from build123d import *

# Parameters (mm, degrees)
F0_W         = 16.3
F0_H         = 8.5
F1_DEPTH     = 22
F2_R         = 5.1
F3_DEPTH     = 22
F4_W         = 3
F4_H         = 12.2
F4_W_2       = 9.2
F5_DEPTH     = 40
F6_R         = 2.5
F7_DEPTH     = 22.001
F6_R_2       = 4.25
F8_DEPTH     = 5
F9_T1_DEPTH  = 85
F9_T3_DEPTH  = 36
F9_T5_DEPTH  = 20
F9_S9_W      = 1
F9_S9_H      = 1
F9_T10_DEPTH = 1
F9_S15_W     = 1
F9_S15_H     = 1
F9_T16_DEPTH = 1
F9_S21_W     = 1
F9_S21_H     = 1
F9_T22_DEPTH = 1
F9_S27_W     = 1
F9_S27_H     = 1
F9_T28_DEPTH = 1
F9_S33_W     = 1
F9_S33_H     = 1
F9_T34_DEPTH = 1
F9_S39_W     = 1
F9_S39_H     = 1
F9_T40_DEPTH = 1
F9_S45_W     = 1
F9_S45_H     = 1
F9_T46_DEPTH = 1
F9_S51_W     = 1
F9_S51_H     = 1
F9_T52_DEPTH = 1


# Not quite as in the source:
# - a fillet or chamfer that OpenCascade refuses, or shapes differently, is made with other operations: its cross-section is extruded or revolved along the edge and cut away or added


with BuildPart() as f1:
    # F0 (on Front) → F1 (new body)
    with BuildSketch(Plane.XZ):
        Polygon((-19, 32), (-6.1, 32), (6.1, 32), (19, 32), (19, 54), (-19, 54), align=None)
        with Locations((0, 43)):
            Rectangle(F0_W, F0_H, mode=Mode.SUBTRACT)
        Polygon((-3.1, -20), (-3.1, 20), (-6.1, 20), (-6.1, 32), (-19, 32), (-19, -33), (19, -33), (19, 32), (6.1, 32), (6.1, 20), (3.1, 20), (3.1, -20), align=None)
    extrude(amount=F1_DEPTH)

    # F2 (on face) → F3 (cut, through all)
    with BuildSketch(Plane.XY.offset(54)):
        with Locations((0, -11)):
            Circle(F2_R)
    extrude(amount=-F3_DEPTH, mode=Mode.SUBTRACT)

    # F4 (on face) → F5 (cut)
    with BuildSketch(Plane.XY.offset(20)):
        with Locations((-4.6, -11.319772105)):
            Rectangle(F4_W, F4_H)
        with Locations((1.5, -11.319772105)):
            Rectangle(F4_W_2, F4_H)
    extrude(amount=-F5_DEPTH, mode=Mode.SUBTRACT)

    # F6 (on face) → F7 (cut, through all)
    with BuildSketch(Plane.XZ.offset(22)):
        with Locations((-13, 49)):
            Circle(F6_R)
        with Locations((13, 49)):
            Circle(F6_R)
        with Locations((-13, -27)):
            Circle(F6_R)
        with Locations((13, -27)):
            Circle(F6_R)
    extrude(amount=-F7_DEPTH, mode=Mode.SUBTRACT)

    # F6 (on face) → F8 (cut)
    with BuildSketch(Plane.XZ.offset(22)):
        with Locations((-13, 49)):
            Circle(F6_R_2)
        with Locations((-13, 49)):
            Circle(F6_R, mode=Mode.SUBTRACT)
        with Locations((13, 49)):
            Circle(F6_R_2)
        with Locations((13, 49)):
            Circle(F6_R, mode=Mode.SUBTRACT)
        with Locations((13, -27)):
            Circle(F6_R_2)
        with Locations((13, -27)):
            Circle(F6_R, mode=Mode.SUBTRACT)
        with Locations((-13, -27)):
            Circle(F6_R_2)
        with Locations((-13, -27)):
            Circle(F6_R, mode=Mode.SUBTRACT)
    extrude(amount=-F8_DEPTH, mode=Mode.SUBTRACT)

    # F9: fillet of radius 1 on 12 edges, made by hand

    # F9_s2 → F9_t1 (cut)
    with BuildSketch(Plane.XY.offset(-32)):
        with BuildLine():
            ThreePointArc((18, -22), (18.7071067812, -21.7071067812), (19, -21))
            Line((19, -21), (19, -22))
            Line((19, -22), (18, -22))
        make_face()
        with BuildLine():
            ThreePointArc((-18, -22), (-18.7071067812, -21.7071067812), (-19, -21))
            Line((-19, -21), (-19, -22))
            Line((-19, -22), (-18, -22))
        make_face()
        with BuildLine():
            ThreePointArc((-18, 0), (-18.7071067812, -0.2928932188), (-19, -1))
            Line((-19, -1), (-19, 0))
            Line((-19, 0), (-18, 0))
        make_face()
        with BuildLine():
            ThreePointArc((18, 0), (18.7071067812, -0.2928932188), (19, -1))
            Line((19, -1), (19, 0))
            Line((19, 0), (18, 0))
        make_face()
    extrude(amount=F9_T1_DEPTH, mode=Mode.SUBTRACT)

    # F9_s4 → F9_t3 (cut)
    with BuildSketch(Plane.YZ.offset(-18)):
        with BuildLine():
            ThreePointArc((-22, 53), (-21.7071067812, 53.7071067812), (-21, 54))
            Line((-21, 54), (-22, 54))
            Line((-22, 54), (-22, 53))
        make_face()
        with BuildLine():
            ThreePointArc((-22, -32), (-21.7071067812, -32.7071067812), (-21, -33))
            Line((-21, -33), (-22, -33))
            Line((-22, -33), (-22, -32))
        make_face()
        with BuildLine():
            ThreePointArc((0, 53), (-0.2928932188, 53.7071067812), (-1, 54))
            Line((-1, 54), (0, 54))
            Line((0, 54), (0, 53))
        make_face()
        with BuildLine():
            ThreePointArc((0, -32), (-0.2928932188, -32.7071067812), (-1, -33))
            Line((-1, -33), (0, -33))
            Line((0, -33), (0, -32))
        make_face()
    extrude(amount=F9_T3_DEPTH, mode=Mode.SUBTRACT)

    # F9_s6 → F9_t5 (cut)
    with BuildSketch(Plane.XZ.offset(1)):
        with BuildLine():
            ThreePointArc((19, -32), (18.7071067812, -32.7071067812), (18, -33))
            Line((18, -33), (19, -33))
            Line((19, -33), (19, -32))
        make_face()
        with BuildLine():
            ThreePointArc((18, 54), (18.7071067812, 53.7071067812), (19, 53))
            Line((19, 53), (19, 54))
            Line((19, 54), (18, 54))
        make_face()
        with BuildLine():
            ThreePointArc((-18, 54), (-18.7071067812, 53.7071067812), (-19, 53))
            Line((-19, 53), (-19, 54))
            Line((-19, 54), (-18, 54))
        make_face()
        with BuildLine():
            ThreePointArc((-19, -32), (-18.7071067812, -32.7071067812), (-18, -33))
            Line((-18, -33), (-19, -33))
            Line((-19, -33), (-19, -32))
        make_face()
    extrude(amount=F9_T5_DEPTH, mode=Mode.SUBTRACT)


with BuildPart() as f9_tool8:
    # F9_s9 → F9_t10 (new body)
    with BuildSketch(Plane.XZ.offset(21)):
        with Locations((18.5, -32.5)):
            Rectangle(F9_S9_W, F9_S9_H)
    extrude(amount=F9_T10_DEPTH)

    # F9_s11 → F9_t12 (revolve, cut)
    with BuildSketch(Plane(origin=(18, -21, -32), x_dir=(-0.7071067812, 0, 0.7071067812), z_dir=(0.7071067812, 0, 0.7071067812))):
        with BuildLine():
            ThreePointArc((0, -1), (1, 0), (0, 1))
            Line((0, 1), (0, -1))
        make_face()
    revolve(axis=Axis((18, -21, -32), (0, -1, 0)), mode=Mode.SUBTRACT)


with BuildPart() as f1_1:
    add(f1.part)

    # F9_t7: cut F9_tool8
    add(f9_tool8.part, mode=Mode.SUBTRACT)


with BuildPart() as f9_tool14:
    # F9_s15 → F9_t16 (new body)
    with BuildSketch(Plane.XY.offset(53)):
        with Locations((18.5, -21.5)):
            Rectangle(F9_S15_W, F9_S15_H)
    extrude(amount=F9_T16_DEPTH)

    # F9_s17 → F9_t18 (revolve, cut)
    with BuildSketch(Plane(origin=(18, -21, 53), x_dir=(-0.7071067812, 0.7071067812, 0), z_dir=(0.7071067812, 0.7071067812, 0))):
        with BuildLine():
            ThreePointArc((0, -1), (1, 0), (0, 1))
            Line((0, 1), (0, -1))
        make_face()
    revolve(axis=Axis((18, -21, 53), (0, 0, 1)), mode=Mode.SUBTRACT)


with BuildPart() as f1_2:
    add(f1_1.part)

    # F9_t13: cut F9_tool14
    add(f9_tool14.part, mode=Mode.SUBTRACT)


with BuildPart() as f9_tool20:
    # F9_s21 → F9_t22 (new body)
    with BuildSketch(Plane.XY.offset(53)):
        with Locations((-18.5, -21.5)):
            Rectangle(F9_S21_W, F9_S21_H)
    extrude(amount=F9_T22_DEPTH)

    # F9_s23 → F9_t24 (revolve, cut)
    with BuildSketch(Plane(origin=(-18, -21, 53), x_dir=(0.7071067812, 0.7071067812, 0), z_dir=(0.7071067812, -0.7071067812, 0))):
        with BuildLine():
            ThreePointArc((0, -1), (1, 0), (0, 1))
            Line((0, 1), (0, -1))
        make_face()
    revolve(axis=Axis((-18, -21, 53), (0, 0, 1)), mode=Mode.SUBTRACT)


with BuildPart() as f1_3:
    add(f1_2.part)

    # F9_t19: cut F9_tool20
    add(f9_tool20.part, mode=Mode.SUBTRACT)


with BuildPart() as f9_tool26:
    # F9_s27 → F9_t28 (new body)
    with BuildSketch(Plane.XZ.offset(21)):
        with Locations((-18.5, -32.5)):
            Rectangle(F9_S27_W, F9_S27_H)
    extrude(amount=F9_T28_DEPTH)

    # F9_s29 → F9_t30 (revolve, cut)
    with BuildSketch(Plane(origin=(-18, -21, -32), x_dir=(0.7071067812, 0, 0.7071067812), z_dir=(0.7071067812, 0, -0.7071067812))):
        with BuildLine():
            ThreePointArc((0, -1), (1, 0), (0, 1))
            Line((0, 1), (0, -1))
        make_face()
    revolve(axis=Axis((-18, -21, -32), (0, -1, 0)), mode=Mode.SUBTRACT)


with BuildPart() as f1_4:
    add(f1_3.part)

    # F9_t25: cut F9_tool26
    add(f9_tool26.part, mode=Mode.SUBTRACT)


with BuildPart() as f9_tool32:
    # F9_s33 → F9_t34 (new body)
    with BuildSketch(Plane.XZ.offset(1)):
        with Locations((18.5, -32.5)):
            Rectangle(F9_S33_W, F9_S33_H)
    extrude(amount=-F9_T34_DEPTH)

    # F9_s35 → F9_t36 (revolve, cut)
    with BuildSketch(Plane(origin=(18, -1, -32), x_dir=(-0.7071067812, 0, 0.7071067812), z_dir=(-0.7071067812, 0, -0.7071067812))):
        with BuildLine():
            ThreePointArc((0, -1), (1, 0), (0, 1))
            Line((0, 1), (0, -1))
        make_face()
    revolve(axis=Axis((18, -1, -32), (0, 1, 0)), mode=Mode.SUBTRACT)


with BuildPart() as f1_5:
    add(f1_4.part)

    # F9_t31: cut F9_tool32
    add(f9_tool32.part, mode=Mode.SUBTRACT)


with BuildPart() as f9_tool38:
    # F9_s39 → F9_t40 (new body)
    with BuildSketch(Plane.XZ.offset(1)):
        with Locations((18.5, 53.5)):
            Rectangle(F9_S39_W, F9_S39_H)
    extrude(amount=-F9_T40_DEPTH)

    # F9_s41 → F9_t42 (revolve, cut)
    with BuildSketch(Plane(origin=(18, -1, 53), x_dir=(-0.7071067812, 0, -0.7071067812), z_dir=(0.7071067812, 0, -0.7071067812))):
        with BuildLine():
            ThreePointArc((0, -1), (1, 0), (0, 1))
            Line((0, 1), (0, -1))
        make_face()
    revolve(axis=Axis((18, -1, 53), (0, 1, 0)), mode=Mode.SUBTRACT)


with BuildPart() as f1_6:
    add(f1_5.part)

    # F9_t37: cut F9_tool38
    add(f9_tool38.part, mode=Mode.SUBTRACT)


with BuildPart() as f9_tool44:
    # F9_s45 → F9_t46 (new body)
    with BuildSketch(Plane.XZ.offset(1)):
        with Locations((-18.5, 53.5)):
            Rectangle(F9_S45_W, F9_S45_H)
    extrude(amount=-F9_T46_DEPTH)

    # F9_s47 → F9_t48 (revolve, cut)
    with BuildSketch(Plane(origin=(-18, -1, 53), x_dir=(0.7071067812, 0, -0.7071067812), z_dir=(0.7071067812, 0, 0.7071067812))):
        with BuildLine():
            ThreePointArc((0, -1), (1, 0), (0, 1))
            Line((0, 1), (0, -1))
        make_face()
    revolve(axis=Axis((-18, -1, 53), (0, 1, 0)), mode=Mode.SUBTRACT)


with BuildPart() as f1_7:
    add(f1_6.part)

    # F9_t43: cut F9_tool44
    add(f9_tool44.part, mode=Mode.SUBTRACT)


with BuildPart() as f9_tool50:
    # F9_s51 → F9_t52 (new body)
    with BuildSketch(Plane.XZ.offset(1)):
        with Locations((-18.5, -32.5)):
            Rectangle(F9_S51_W, F9_S51_H)
    extrude(amount=-F9_T52_DEPTH)

    # F9_s53 → F9_t54 (revolve, cut)
    with BuildSketch(Plane(origin=(-18, -1, -32), x_dir=(0.7071067812, 0, 0.7071067812), z_dir=(-0.7071067812, 0, 0.7071067812))):
        with BuildLine():
            ThreePointArc((0, -1), (1, 0), (0, 1))
            Line((0, 1), (0, -1))
        make_face()
    revolve(axis=Axis((-18, -1, -32), (0, 1, 0)), mode=Mode.SUBTRACT)


with BuildPart() as f1_8:
    add(f1_7.part)

    # F9_t49: cut F9_tool50
    add(f9_tool50.part, mode=Mode.SUBTRACT)


solid = f1_8.part
Design review of the part built by this model. Coordinates are the model's own, in mm. A direction names the side the tool comes from. Round coordinates to 2 decimals unless told otherwise and drop trailing zeros. Write each loop counter-clockwise with the first axis right and the second up, starting at its lowest first coordinate (ties: lowest second). Pieces come first, ordered by that corner, then holes. Notation, with made-up numbers: (-40, 69.25) -> (-10, 69.25) arc R24 ccw to (-10, 80.25) -> close; hole circle Ø9 at (3, 69). An arc over 180 degrees is marked (long way). One line per question, with ' | ' between items.
(1) Take a section at B-B, the plane z = 49. State the section outline as (x, y) points, and give its area (3 significant figures).
Result sheet:
outline: (-19, -21) arc R1 ccw to (-18, -22) -> (-17.25, -22) -> (-17.25, -17) -> (-15.5, -17) -> (-15.5, 0) -> (-18, 0) arc R1 ccw to (-19, -1) -> close; (-10.5, -17) -> (-8.75, -17) -> (-8.75, -22) -> (8.75, -22) -> (8.75, -17) -> (10.5, -17) -> (10.5, 0) -> (-10.5, 0) -> close; (15.5, -17) -> (17.25, -17) -> (17.25, -22) -> (18, -22) arc R1 ccw to (19, -21) -> (19, -1) arc R1 ccw to (18, 0) -> (15.5, 0) -> close; hole circle Ø10.2 at (0, -11) | area: 498 mm2
(2) Take a section at C-C, the plane y = -11. State the section outline as (x, z) points.
Result sheet:
outline: (-19, -32) arc R1 ccw to (-18, -33) -> (18, -33) arc R1 ccw to (19, -32) -> (19, 53) arc R1 ccw to (18, 54) -> (5.1, 54) -> (5.1, 47.25) -> (8.15, 47.25) -> (8.15, 38.75) -> (5.1, 38.75) -> (5.1, 32) -> (6.1, 32) -> (6.1, -20) -> (-6.1, -20) -> (-6.1, 32) -> (-5.1, 32) -> (-5.1, 38.75) -> (-8.15, 38.75) -> (-8.15, 47.25) -> (-5.1, 47.25) -> (-5.1, 54) -> (-18, 54) arc R1 ccw to (-19, 53) -> close; hole circle Ø5 at (-13, -27); hole circle Ø5 at (-13, 49); hole circle Ø5 at (13, -27); hole circle Ø5 at (13, 49)
(3) Take a section at A-A, the plane x = 0. State the section outline as (y, z) points.
Result sheet:
outline: (-22, -32) arc R1 ccw to (-21, -33) -> (-1, -33) arc R1 ccw to (0, -32) -> (0, -20) -> (-22, -20) -> close; (-22, 32) -> (-16.1, 32) -> (-16.1, 38.75) -> (-22, 38.75) -> close; (-22, 47.25) -> (-16.1, 47.25) -> (-16.1, 54) -> (-21, 54) arc R1 ccw to (-22, 53) -> close; (-5.9, 32) -> (0, 32) -> (0, 38.75) -> (-5.9, 38.75) -> close; (-5.9, 47.25) -> (0, 47.25) -> (0, 53) arc R1 ccw to (-1, 54) -> (-5.9, 54) -> close
(4) Machinability: for faces 4 (the flat face through (-11, -17, -29)), 5 (the flat face through (0, -11, -20)), 6 (the flat face through (-8.15, -11, 43)), which of the approach directions +Z, -Z, +X, -X, +Y, -Y give a long, thin tool a straight path to every point of the face, cutting with its end or side? Answer none if there is none.
Result sheet:
face 4: -Y | face 5: none | face 6: +Y, -Y
(5) Take a section at D-D, the plane x = -7. State the section outline as (y, z) points.
Result sheet:
outline: (-22, -32) arc R1 ccw to (-21, -33) -> (-1, -33) arc R1 ccw to (0, -32) -> (0, 38.75) -> (-22, 38.75) -> close; (-22, 47.25) -> (0, 47.25) -> (0, 53) arc R1 ccw to (-1, 54) -> (-21, 54) arc R1 ccw to (-22, 53) -> close
(6) Insertion check: P1, Ø8, axis at x = 0, y = -11, coming from the +Z side; P2, Ø4, axis at x = 12, z = 49, coming from the -Y side. Each pin has a flat end and moves straight along its axis. Give the tip position at first contact, or say it passes through.
Result sheet:
P1: z = -20 | P2: y = -17
(7) Draft analysis for pull direction Y (two halves, no side actions). For faces 1 (the cylindrical face through (12.46, -8.62, 46.56)), 2 (the flat face through (-4, 0, 11)), 3 (the flat face through (6.1, -11, 12)), state which applies: released by +Y, released by -Y, zero draft, split by the parting line, or undercut.
Result sheet:
face 1: zero draft | face 2: released by +Y | face 3: undercut
(8) Wall thickness on line 1 (X direction, y = -19.05, z = 49); line 2 (Z direction, x = -13, y = -19.15); line 3 (Z direction, x = -1, y = -17.25): over which ranges is each line inside the solid? List them lowest first. Write a range as [from, to].
Result sheet:
line 1: [-19, -17.25], [-8.75, 8.75], [17.25, 19] | line 2: [-33, -31.25], [-22.75, 44.75], [53.25, 54] | line 3: [-33, -20], [32, 38.75], [47.25, 54]
